Read the model definition and answer for the solid it produces. Units are mm, in the model's axes. A direction names the side the tool comes from. Coordinates: 2 decimals unless noted, no trailing zeros. Order: outer loops, then holes, each group sorted by start corner. A loop starts at its lowest first (then second) coordinate and runs counter-clockwise, first axis right, second up. Notation, with made-up numbers: (47.25, -8) -> (98.25, -8) arc R17 cw to (98.25, 19) -> close; hole circle Ø1 at (62.5, 32). An arc over 180 degrees is marked (long way). Answer in a Markdown table with one row per item.
from build123d import *

# Parameters (mm, degrees)
SKETCH_R     = 2.75
PAD_DEPTH    = 2
SKETCH001_R  = 1.5
PAD001_DEPTH = 25
FILLET_R     = 0.5


with BuildPart() as part:
    # Sketch → Pad (new body)
    with BuildSketch(Plane.XY):
        Circle(SKETCH_R)
    extrude(amount=PAD_DEPTH)

    # Sketch001 → Pad001 (new body)
    with BuildSketch(Plane.XY.offset(2)):
        Circle(SKETCH001_R)
    extrude(amount=PAD001_DEPTH)

    # Fillet
    fillet_edges = [part.edges().sort_by_distance(p)[0] for p in [
        (-2.75, 0, 0),
    ]]
    fillet(fillet_edges, radius=FILLET_R)


solid = part.part
Q1. For faces 1 (the face through (-1.5, 0.07, 14.32)), 2 (the face through (-0.596, -2.685, 1.24)), determine the directions among +Z, -Z, +X, -X, +Y, -Y from which every point of the face is accessible in a straight line to the end or side of a thin tool.
Outcome:
| item | result |
|---|---|
| face 1 | +Z |
| face 2 | +Z, -Z |
Q2. The part is cut by section C-C (z = 17.5). Write down the section's boundary in (x, y), then the cut area to 3 significant figures.
Outcome:
| item | result |
|---|---|
| outline | circle Ø3 at (0, 0) |
| area | 7.07 mm² |
Q3. Consider line 1 (Z direction, x = -1.7, y = 0.1); line 2 (Y direction, x = -0.1, z = 15.5); line 3 (Y direction, x = -1.2, z = 6.5). Determine where each line is inside the solid, lowest interval first.
Outcome:
| item | result |
|---|---|
| line 1 | 0 to 2 |
| line 2 | -1.5 to 1.5 |
| line 3 | -0.9 to 0.9 |
Q4. The part is cut by section A-A (y = 0). Write down the section's boundary in (x, z).
Outcome:
| item | result |
|---|---|
| outline | (-2.75, 0.5) arc R0.5 ccw to (-2.25, 0) -> (2.25, 0) arc R0.5 ccw to (2.75, 0.5) -> (2.75, 2) -> (1.5, 2) -> (1.5, 27) -> (-1.5, 27) -> (-1.5, 2) -> (-2.75, 2) -> close |
Q5. Given pin 1 (1.5 mm diameter, centred on x = 1.5, z = 4.5, fed in from +Y); pin 2 (1 mm diameter, centred on y = -1, z = 12, fed in from -X); pin 3 (1.5 mm diameter, centred on y = -0.5, z = 11, fed in from +X), each flat-ended and moving along its own axis, determine where each tip first touches the part or whether it passes through.
Outcome:
| item | result |
|---|---|
| pin 1 | y = 1.3 |
| pin 2 | x = -1.41 |
| pin 3 | x = 1.5 |
